Here's how the part is built. I have some questions about the finished solid (model axes, mm). A direction names the side the tool comes from. Round coordinates to 2 decimals unless told otherwise and drop trailing zeros. Order: outer loops, then holes, each group sorted by start corner. A loop starts at its lowest first (then second) coordinate and runs counter-clockwise, first axis right, second up. Notation, with made-up numbers: (56, -14.75) -> (98, -14.75) arc R25 ccw to (98, 8.25) -> close; hole circle Ø7 at (78, 79.25). An arc over 180 degrees is marked (long way). Use a Markdown table: item, result. Add a question column.
(1) I want a section at D-D, the plane x = -300.5. Please give me the cut outline in (y, z).
(2) I'm going to push flat-ended pins straight in: P1, Ø2, axis at y = -6, z = 1, coming from the +X side; P2, Ø2, axis at y = 15, z = 1.5, coming from the +X side; P3, Ø1.2, axis at y = 9, z = 1.5, coming from the -X side. Where does each tip first touch, or does it pass through?
(3) On a 3-axis mill with a long thin cutter (end or side, diameter ignored), from which of +Z, -Z, +X, -X, +Y, -Y can I reach the whole of each face in a straight line? I mean faces 1 (the face through (-5, 31, 4)), 2 (the face through (98.47, 29.32, 2.03)). Say none if no direction works.
(4) I want a section at C-C, the plane z = 3.4. Give the number of separate pieces and of enclosed holes in the cut face, then the cut area to 3 significant figures.
(5) Thinking about a two-plate mould opening in Y: for faces 3 (the face through (-5, 31, 0)), 4 (the face through (-275.247, -31.077, 1.972)), 5 (the face through (5.83, 29.32, 2.03)), which applies, pulls with the +Y half, pulls with the -Y half, needs draft (parallel to the pull), parting line crosses it, or undercut?
(6) I want a section at B-B, the plane x = 85. Please give me the cut outline in (y, z).
(7) I want a section at A-A, the plane x = -98.5. Please give me the cut outline in (y, z), then the cut area to 3 significant figures.
(8) If I drill on probe 1 along Y at (x, z) = (-74, 3.45); probe 2 along Y at (x, z) = (-257, 0.4); probe 3 along X at (y, z) = (14, 1.3), over which ranges is the centre line in solid material (lowest first)?
from build123d import *

# Parameters (mm, degrees)
SKETCH_1_R          = 3.25
EXTRUDE_1_DEPTH     = 4
HOLE_WIZARD_M32_D   = 3.4
HOLE_WIZARD_M52_D   = 5.5
CUT_EXTRUDE_3_DEPTH = 353.903669576
FILLET_2_R          = 10
FILLET_3_R          = 10
HOLE_WIZARD_M31_D   = 3.4
FILLET_4_R          = 8


with BuildPart() as part:
    # Эскиз1 → Бобышка-Вытянуть1 (new body)
    with BuildSketch(Plane.XY):
        with BuildLine():
            Line((-349.818316726, 27.672449915), (-342.910885265, -16.303620822))
            Line((-342.910885265, -16.303620822), (-211.481081006, -45))
            Line((-211.481081006, -45), (211.481081006, -45))
            Line((211.481081006, -45), (342.910885265, -16.303620822))
            Line((342.910885265, -16.303620822), (349.818316726, 27.672449915))
            ThreePointArc((349.818316726, 27.672449915), (346.399852001, 39.749019149), (335, 45))
            Line((335, 45), (-335, 45))
            ThreePointArc((-335, 45), (-346.399852001, 39.749019149), (-349.818316726, 27.672449915))
        make_face()
        with Locations((-335, -10.635315981)):
            Circle(SKETCH_1_R, mode=Mode.SUBTRACT)
        with Locations(Location((335, -10.635315981, 0), (0, 0, 180))):
            Circle(SKETCH_1_R, mode=Mode.SUBTRACT)
    extrude(amount=EXTRUDE_1_DEPTH)

    # Отверстие с зазором M32 (through all)
    with Locations(Plane.XY.offset(4)):
        with Locations((-335, 40), (-345, 30), (-335, 20), (-325, 30), (325, 30), (335, 40), (345, 30), (335, 20)):
            Hole(HOLE_WIZARD_M32_D / 2)

    # Отверстие с зазором M52 (through all)
    with Locations(Plane(origin=(0, 0, 0), x_dir=(-1, 0, 0), z_dir=(0, 0, -1))):
        with Locations((55, -6), (238.23, 10.84)):
            Hole(HOLE_WIZARD_M52_D / 2)

    # Эскиз10 → Вырез-Вытянуть3 (cut, through all)
    with BuildSketch(Plane.XY.offset(4)):
        with BuildLine():
            Line((-286.571319769, 35), (-242.571319769, 35))
            ThreePointArc((-242.571319769, 35), (-246.739453064, 3.999106889), (-245.818518827, -27.267178292))
            Line((-245.818518827, -27.267178292), (-286.571319769, -18.369213063))
            Line((-286.571319769, -18.369213063), (-286.571319769, 35))
        make_face()
        with BuildLine():
            Line((-226.671925486, 35), (-46.587816989, 35))
            Line((-46.587816989, 35), (-64.032014151, -1.707830342))
            ThreePointArc((-64.032014151, -1.707830342), (-64.961194769, -6.880112935), (-63.13950341, -11.809344562))
            Line((-63.13950341, -11.809344562), (-46.587816989, -35))
            Line((-46.587816989, -35), (-210.402090952, -35))
            Line((-210.402090952, -35), (-229.752534006, -30.775024894))
            ThreePointArc((-229.752534006, -30.775024894), (-231.306735573, 2.257420391), (-226.671925486, 35))
        make_face()
        Polygon((286.571319769, 35), (286.571319769, -18.369213063), (210.402090952, -34), (210.402090952, 35), align=None)
        Polygon((200.402090952, 35), (126.145146633, 35), (63.036502818, 22.049392771), (63.036502818, -35), (137.293447136, -35), (200.402090952, -22.049392771), align=None)
        Polygon((-29.597909048, 22.049392771), (-29.597909048, -35), (-10.072140997, -35), (53.036502818, -22.049392771), (53.036502818, 35), (33.510734767, 35), align=None)
    extrude(amount=-CUT_EXTRUDE_3_DEPTH, mode=Mode.SUBTRACT)

    # Скругление2
    fillet_2_edges = [part.edges().sort_by_distance(p)[0] for p in [
        (210.402090952, 35, 2),
        (286.571319769, 35, 2),
        (286.571319769, -18.369213063, 2),
        (210.402090952, -34, 2),
        (-210.402090952, -35, 2),
        (-229.752534006, -30.775024894, 2),
        (-226.671925486, 35, 2),
        (-46.587816989, 35, 2),
        (342.910885265, -16.303620822, 2),
        (211.481081006, -45, 2),
        (-211.481081006, -45, 2),
        (-342.910885265, -16.303620822, 2),
        (-286.571319769, -18.369213063, 2),
        (-286.571319769, 35, 2),
        (-242.571319769, 35, 2),
        (-245.818518827, -27.267178292, 2),
    ]]
    fillet(fillet_2_edges, radius=FILLET_2_R)

    # Скругление3
    fillet_3_edges = [part.edges().sort_by_distance(p)[0] for p in [
        (63.036502818, 22.049392771, 2),
        (126.145146633, 35, 2),
        (200.402090952, 35, 2),
        (200.402090952, -22.049392771, 2),
        (137.293447136, -35, 2),
        (63.036502818, -35, 2),
        (33.510734767, 35, 2),
        (53.036502818, 35, 2),
        (53.036502818, -22.049392771, 2),
        (-10.072140997, -35, 2),
        (-29.597909048, -35, 2),
        (-29.597909048, 22.049392771, 2),
    ]]
    fillet(fillet_3_edges, radius=FILLET_3_R)

    # Отверстие с зазором M31 (through all)
    with Locations(Plane.XY.offset(4)):
        with Locations((-34.597909048, 28), (-34.597909048, -27), (205.402090952, -27), (205.402090952, 28), (291.571319769, 33), (291.6163356, -2), (-291.6163356, -2), (-291.571319769, 33), (58.036502818, 28), (58.036502818, -27)):
            Hole(HOLE_WIZARD_M31_D / 2)

    # Скругление4
    fillet_4_edges = [part.edges().sort_by_distance(p)[0] for p in [
        (-46.587816989, -35, 2),
    ]]
    fillet(fillet_4_edges, radius=FILLET_4_R)


solid = part.part
Taken from the geometry:
| question | item | result |
|---|---|---|
| 1 | outline | (-25.56, 0) -> (45, 0) -> (45, 4) -> (-25.56, 4) -> close |
| 2 | P1 | stops at x = 344.69 |
| 2 | P2 | stops at x = 347.98 |
| 2 | P3 | stops at x = -346.98 |
| 3 | face 1 | +Z, +X, -X, +Y, -Y |
| 3 | face 2 | +Z, -Z |
| 4 | separate pieces | 1 |
| 4 | enclosed holes | 27 |
| 4 | area | 25,700 mm2 |
| 5 | face 3 | needs draft |
| 5 | face 4 | pulls with the -Y half |
| 5 | face 5 | undercut |
| 6 | outline | (-45, 0) -> (-35, 0) -> (-35, 4) -> (-45, 4) -> close; (26.56, 0) -> (45, 0) -> (45, 4) -> (26.56, 4) -> close |
| 7 | outline | (-45, 0) -> (-35, 0) -> (-35, 4) -> (-45, 4) -> close; (35, 0) -> (45, 0) -> (45, 4) -> (35, 4) -> close |
| 7 | area | 80.0 mm2 |
| 8 | probe 1 | y = -45 to -35, 35 to 45 |
| 8 | probe 2 | y = -35.06 to -24.63, 35 to 45 |
| 8 | probe 3 | x = -347.67 to -286.57, -245.96 to -230.36, -56.57 to -29.6, 53.04 to 63.04, 200.4 to 210.4, 286.57 to 347.67 |
